from build123d import *

# Parameters (mm, degrees)
F0_W          = 2.54
F0_H          = 2.54
F1_DEPTH      = 5.08
F1_DEPTH_BACK = 5.08
F0_W_2        = 12.7
F2_DEPTH      = 25.4
F2_DEPTH_BACK = 25.4
F3_R          = 2.54


with BuildPart() as f1:
    # F0 (on Front) → F1 (new body, two sides)
    with BuildSketch(Plane.XZ) as f1_sk:
        Polygon((-2.54, 111.76), (0, 111.76), (0, 121.92), (-15.24, 121.92), (-22.86, 125.73), (-22.86, 122.8901936686), (-18.4033727053, 120.6618800212), (-15.8396126628, 119.38), (-14.30558227, 119.38), (-2.54, 119.38), align=None)
        Polygon((-15.2376033366, -121.92), (0, -121.92), (0, 109.22), (-2.54, 109.22), (-2.54, -119.38), (-15.2376033366, -119.38), align=None)
        with Locations((-1.27, 110.49)):
            Rectangle(F0_W, F0_H)
        Polygon((-15.9520190209, 117.9121956229), (-14.30558227, 119.38), (-15.8396126628, 119.38), (-18.4033727053, 120.6618800212), align=None)
    extrude(amount=F1_DEPTH)
    extrude(f1_sk.sketch, amount=-F1_DEPTH_BACK)

    # F0 (on Front) → F2 (join, two sides)
    with BuildSketch(Plane.XZ) as f2_sk:
        with Locations((-1.27, 110.49)):
            Rectangle(F0_W, F0_H)
        with Locations((-8.89, 110.49)):
            Rectangle(F0_W_2, F0_H)
    extrude(amount=F2_DEPTH)
    extrude(f2_sk.sketch, amount=-F2_DEPTH_BACK)

    # F3
    f3_edges = [f1.edges().sort_by_distance(p)[0] for p in [
        (-2.54, 0, -119.38),
    ]]
    fillet(f3_edges, radius=F3_R)


solid = f1.part
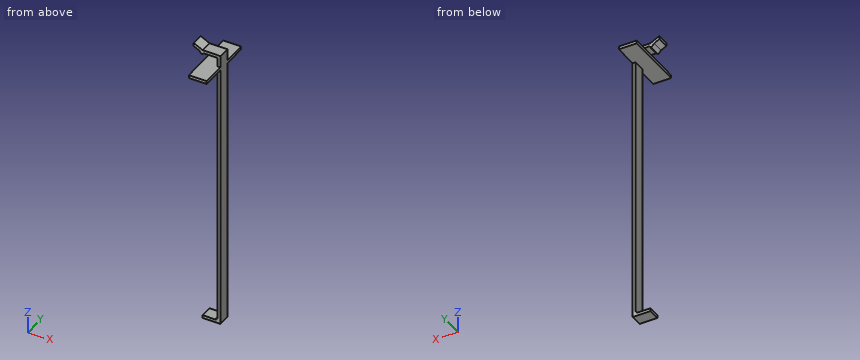
Model file for the job. Use its own axes, mm. Give positions to 0.01 mm unless a question says otherwise; leave off trailing zeros. Write each loop counter-clockwise with the first axis right and the second up, starting at its lowest first coordinate (ties: lowest second). Pieces come first, ordered by that corner, then holes. Notation, with made-up numbers: M 85,27 L 136,27 A9 cw 136,39 Z; hole C 86,52 d9. An arc over 180 degrees is marked long. One line per item, written item: value. Start each with the question number.
Q1. Saw through at A-A, the plane x = -8.5. Write the cut outline in (y, z).
Q2. Saw through at D-D, the plane y = -13. Write the cut outline in (x, z), plus the area to 3 significant figures.
Q3. Saw through at B-B, the plane y = 1.5. Write the cut outline in (x, z).
Q4. Drop flat-ended pins along their axis: pin 1 Ø11 at (y, z) = (-0.5, -48.5) entering from -X; pin 2 Ø4.5 at (x, z) = (-4, 14) entering from -Y; pin 3 Ø11 at (x, y) = (-10, 0.5) entering from +Z. Give the stop position or say it passes through.
Q5. Probe probe 1 along Z at (x, y) = (-12, 4.5); probe 2 along Z at (x, y) = (-11.75, -11); probe 3 along X at (y, z) = (5, -78). List the from-to ranges inside material, lowest first. Write a range as [from, to].
Q6. Saw through at C-C, the plane z = 5.5. Write the cut outline in (x, y).
Output values:
1. outline: M -25.4,109.22 L 25.4,109.22 L 25.4,111.76 L -25.4,111.76 Z; M -5.08,-121.92 L 5.08,-121.92 L 5.08,-119.38 L -5.08,-119.38 Z; M -5.08,119.38 L 5.08,119.38 L 5.08,121.92 L -5.08,121.92 Z
2. outline: M -15.24,109.22 L 0,109.22 L 0,111.76 L -15.24,111.76 Z
2. area: 38.7 mm²
3. outline: M -22.86,122.89 L -18.4,120.66 L -15.95,117.91 L -14.31,119.38 L -2.54,119.38 L -2.54,111.76 L -15.24,111.76 L -15.24,109.22 L -2.54,109.22 L -2.54,-116.84 A2.54 cw -5.08,-119.38 L -15.24,-119.38 L -15.24,-121.92 L 0,-121.92 L 0,121.92 L -15.24,121.92 L -22.86,125.73 Z
4. pin 1: stops at x = -2.54
4. pin 2: stops at y = -5.08
4. pin 3: stops at z = 122.05
5. probe 1: z = [-121.92, -119.38], [109.22, 111.76], [119.38, 121.92]
5. probe 2: z = [109.22, 111.76]
5. probe 3: x = [-2.54, 0]
6. outline: M -2.54,-5.08 L 0,-5.08 L 0,5.08 L -2.54,5.08 Z
